Can you work these out from the model? Positions are in its coordinate system, mm. Face numbers are marked on the shaded views. A direction names the side the tool comes from. Coordinates: 2 decimals unless noted, no trailing zeros. Order: outer loops, then holes, each group sorted by start corner. A loop starts at its lowest first (then second) coordinate and runs counter-clockwise, first axis right, second up. Notation, with made-up numbers: (62, -28) - (94, -28) arc R20 cw to (94, 9) - close; hole circle Ø1 at (81, -22.75). An arc over 180 degrees is marked (long way). Return JSON: item names as keys, results as strings. Group by question number.
1) For pin 1 Ø4 at (x, y) = (-15.5, 16) entering from -Z; pin 2 Ø5 at (x, y) = (-22.5, -20) entering from +Z; pin 3 Ø7.5 at (y, z) = (-12, 15.5) entering from +X, each with a flat end and sliding along its axis, tell me the tip position at first contact or that it passes through.
2) Imagine slicing it at B-B (x = -6). Write out the boundary of the cut face in (y, z).
3) Imagine slicing it at C-C (z = 19.5). Write out the boundary of the cut face in (x, y), and give its area (3 significant figures).
4) If we mould it in two halves opening along X, with no side actions, what happens to the marked faces 1, 2, 3 and 4? For each: pulls with the +X half, pulls with the -X half, needs draft (parallel to the pull), parting line crosses it, or undercut.
5) Which directions (+Z, -Z, +X, -X, +Y, -Y) give clear straight access to the entire face, cutting with the end or side of a thin tool? Please do the marked faces 5, 6 and 7.
6) Imagine slicing it at D-D (y = 16). Write out the boundary of the cut face in (x, z), and give its area (3 significant figures).
7) If I drill on line 1 along Z through (x, y) = (-15.5, 19.5); line 2 along Y through (x, z) = (5.5, 15.5); line 3 along Y through (x, z) = (-9, 18.5), over which ranges is the centre line in solid material (lowest first)?
8) Imagine slicing it at A-A (y = 2.5). Write out the boundary of the cut face in (x, z).
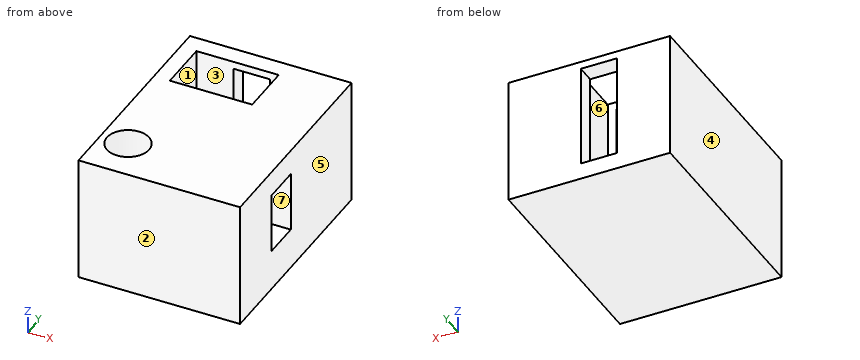
```python
from build123d import *

# Parameters (mm, degrees)
F0_W      = 39.2675818875
F0_H      = 53.094195202
F1_DEPTH  = 30.734
F2_R      = 5.9033693707
F3_DEPTH  = 34.544
F4_R      = 6.9366562731
F5_DEPTH  = 29.21
F6_R      = 5.137322698
F7_DEPTH  = 25.4
F8_W      = 9.2991222627
F8_H      = 14.6318394691
F9_DEPTH  = 25.4
F10_W     = 8.8133979589
F10_H     = 24.9259229749
F11_DEPTH = 25.4
F12_W     = 20.0094743632
F12_H     = 12.6438736916
F13_DEPTH = 25.4


with BuildPart() as f1:
    # F0 (on Top) → F1 (new body)
    with BuildSketch(Plane.XY):
        with Locations((-9.2177423649, -5.0697578117)):
            Rectangle(F0_W, F0_H)
    extrude(amount=F1_DEPTH)

    # F2 (on face) → F3 (join)
    with BuildSketch(Plane(origin=(0, 21.4773397893, 0), x_dir=(-1, 0, 0), z_dir=(0, 1, 0))):
        with Locations((0, 21.7559281737)):
            Circle(F2_R)
    extrude(amount=-F3_DEPTH)

    # F4 (on face) → F5 (join)
    with BuildSketch(Plane(origin=(0, 21.4773397893, 0), x_dir=(-1, 0, 0), z_dir=(0, 1, 0))):
        with Locations((0, 17.7725534886)):
            Circle(F4_R)
    extrude(amount=-F5_DEPTH)

    # F6 (on face) → F7 (cut)
    with BuildSketch(Plane.XY.offset(30.734)):
        with Locations((-22.2064536065, -21.0470482707)):
            Circle(F6_R)
    extrude(amount=-F7_DEPTH, mode=Mode.SUBTRACT)

    # F8 (on face) → F9 (cut)
    with BuildSketch(Plane.YZ.offset(10.4160485789)):
        with Locations((-12.1103653219, 17.2777241096)):
            Rectangle(F8_W, F8_H)
    extrude(amount=-F9_DEPTH, mode=Mode.SUBTRACT)

    # F10 (on face) → F11 (cut)
    with BuildSketch(Plane(origin=(0, 21.4773397893, 0), x_dir=(-1, 0, 0), z_dir=(0, 1, 0))):
        with Locations((11.5594444796, 16.4570594206)):
            Rectangle(F10_W, F10_H)
    extrude(amount=-F11_DEPTH, mode=Mode.SUBTRACT)

    # F12 (on face) → F13 (cut)
    with BuildSketch(Plane.XY.offset(30.734)):
        with Locations((-14.995142119, 10.6841661036)):
            Rectangle(F12_W, F12_H)
    extrude(amount=-F13_DEPTH, mode=Mode.SUBTRACT)


solid = f1.part
```
Calculated:
{
 "1": {"pin 1": "z = 0", "pin 2": "z = 5.33", "pin 3": "x = -14.98"},
 "2": {"outline": "(-31.62, 0) - (21.48, 0) - (21.48, 30.73) - (17.01, 30.73) - (17.01, 5.33) - (4.36, 5.33) - (4.36, 30.73) - (-31.62, 30.73) - close; hole (-16.76, 9.96) - (-7.46, 9.96) - (-7.46, 24.59) - (-16.76, 24.59) - close"},
 "3": {"outline": "(-28.85, -31.62) - (10.42, -31.62) - (10.42, -16.76) - (-14.98, -16.76) - (-14.98, -7.46) - (10.42, -7.46) - (10.42, 21.48) - (-7.15, 21.48) - (-7.15, 17.01) - (-4.99, 17.01) - (-4.99, 4.36) - (-7.15, 4.36) - (-7.15, -3.92) - (-15.97, -3.92) - (-15.97, 4.36) - (-25, 4.36) - (-25, 17.01) - (-15.97, 17.01) - (-15.97, 21.48) - (-28.85, 21.48) - close; hole circle Ø10.27 at (-22.21, -21.05)", "area": "1,400 mm2"},
 "4": {"face 1": "undercut", "face 2": "needs draft", "face 3": "undercut", "face 4": "pulls with the -X half"},
 "5": {"face 5": "+Z, -Z, +X, +Y, -Y", "face 6": "+Z", "face 7": "+X"},
 "6": {"outline": "(-28.85, 0) - (10.42, 0) - (10.42, 30.73) - (-4.99, 30.73) - (-4.99, 5.33) - (-7.15, 5.33) - (-7.15, 3.99) - (-15.97, 3.99) - (-15.97, 5.33) - (-25, 5.33) - (-25, 30.73) - (-28.85, 30.73) - close", "area": "687 mm2"},
 "7": {"line 1": "0 to 3.99, 28.92 to 30.73", "line 2": "-31.62 to -16.76, -7.46 to 21.48", "line 3": "-31.62 to -16.76, -7.46 to -3.92"},
 "8": {"outline": "(-28.85, 0) - (10.42, 0) - (10.42, 30.73) - (-28.85, 30.73) - close; hole (-15.97, 3.99) - (-7.15, 3.99) - (-7.15, 28.92) - (-15.97, 28.92) - close"}
}
